from build123d import *
from OCP.BRepFilletAPI import BRepFilletAPI_MakeChamfer

# Parameters (mm, degrees)
CHAMFER1_SIZE  = 0.2
CHAMFER1_SIZE2 = 0.546410162


with BuildPart() as part:
    # Sketch2 → Revolve1 (revolve)
    with BuildSketch(Plane(origin=(0, 0, 0), x_dir=(0, 0, -1), z_dir=(1, 0, 0))):
        Polygon((-19, 0), (-19, 10), (-18, 10), (-18, 15), (-19, 15), (-19, 18), (-18.5, 18), (-18.5, 19), (-19, 19), (-19, 22), (-18.5, 22), (-18.5, 23), (-19, 23), (-19, 38), (-18, 38), (-18, 36), (-17, 36), (-16, 37), (-12, 37), (-12, 36), (-7.5, 33.401923789), (-7.5, 30.401923789), (-5, 30.401923789), (-5, 29.401923789), (-7.5, 29.401923789), (-7.5, 26.401923789), (0, 26.401923789), (0, 0), align=None)
    revolve(axis=Axis((0, 26.401923789, 0), (0, -1, 0)))

    # Chamfer1: one chamfer whose edges measure the first distance from different faces: ONE call of the kernel's chamfer builder (chamfer() names one face for all edges)
    chamfer1_edges_1 = [part.edges().sort_by_distance(p)[0] for p in [
        (0, 30.401923789, -5),
        (0, 37, -12),
        (0, 38, -18),
        (0, 38, -19),
        (0, 23, -19),
        (0, 22, -19),
        (0, 19, -19),
        (0, 18, -19),
        (0, 15, -19),
        (0, 10, -19),
        (0, 0, -19),
    ]]
    chamfer1_edges_2 = [part.edges().sort_by_distance(p)[0] for p in [
        (0, 33.401923789, -7.5),
    ]]
    chamfer1_side_2 = [part.faces().sort_by_distance(p)[0] for p in [
        (0, 34.700961894, -9.75),
    ]]
    chamfer1 = BRepFilletAPI_MakeChamfer(part.part.solid().wrapped)
    for e in chamfer1_edges_1:
        chamfer1.Add(CHAMFER1_SIZE, e.wrapped)
    for e in chamfer1_edges_2:
        chamfer1.Add(CHAMFER1_SIZE, CHAMFER1_SIZE2, e.wrapped, chamfer1_side_2[0].wrapped)  # the first distance lies on this face
    add(Compound.cast(chamfer1.Shape()), mode=Mode.REPLACE)


solid = part.part
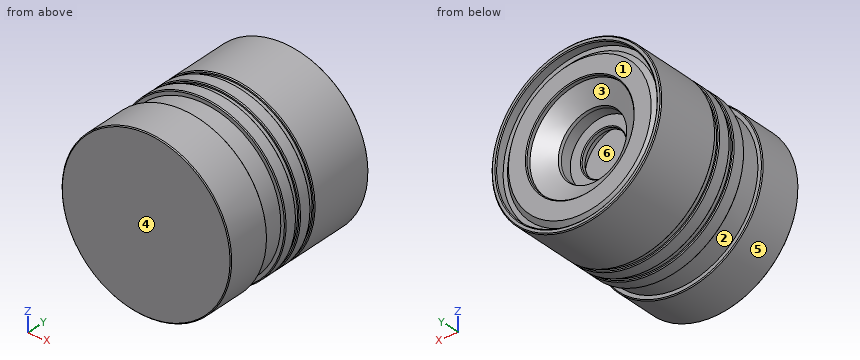
Geometry check sheet. Reference: the model listing, model coordinates, mm. Face numbers are marked on the shaded views. A direction names the side the tool comes from. Give positions to 0.01 mm unless a question says otherwise; leave off trailing zeros. Write each loop counter-clockwise with the first axis right and the second up, starting at its lowest first coordinate (ties: lowest second). Pieces come first, ordered by that corner, then holes. Notation, with made-up numbers: (51.25, -19) - (73.25, -19) arc R15 ccw to (73.25, 9) - close; hole circle Ø1 at (35, 67.25). An arc over 180 degrees is marked (long way). Put each result on its own line as item: value.
1. Draft check along Z on the marked faces 1, 2, 3 and 4. Enter one of: +Z half, -Z half, draft (parallel to the pull), parting line (faces both ways), or undercut.
Ans:
face 1: undercut
face 2: parting line
face 3: undercut
face 4: draft
2. Go/stop test with flat-tipped pins: pin 1 (1 mm diameter, centred on x = -1, z = 9, fed in from +Y); pin 2 (12 mm diameter, centred on x = 0, z = 0, fed in from +Y); pin 3 (2 mm diameter, centred on x = -2.5, y = 26, fed in from +Z). Record where each tip stops, or that it passes through.
Ans:
pin 1: stops at y = 34.59
pin 2: stops at y = 30.4
pin 3: stops at z = 18.94
3. Sectioned sample at A-A, the plane y = 6.5. Enter the section's corners in (x, z).
Ans:
outline: circle Ø38 at (0, 0)
4. Set-up check for the marked faces 5 and 6: record each of +Z, -Z, +X, -X, +Y, -Y from which the full face is reachable in a straight line by a thin tool's end or side.
Ans:
face 5: +Y, -Y
face 6: none
5. Sectioned sample at B-B, the plane y = 13. Enter the section's corners in (x, z).
Ans:
outline: circle Ø36 at (0, 0)
6. Thickness scan on line 1 (X direction, y = 29.95, z = 0); line 2 (X direction, y = 36.5, z = 5); line 3 (X direction, y = 32, z = 0). Record the ranges inside material, lowest first.
Ans:
line 1: x = -19 to -5, 5 to 19
line 2: x = -18.33 to -17.29, -15.72 to -10.91, 10.91 to 15.72, 17.29 to 18.33
line 3: x = -19 to -7.5, 7.5 to 19
